Design review of the part built by this model. Coordinates are the model's own, in mm. A direction names the side the tool comes from. Coordinates: 2 decimals unless noted, no trailing zeros. Write each loop counter-clockwise with the first axis right and the second up, starting at its lowest first coordinate (ties: lowest second). Pieces come first, ordered by that corner, then holes.
```python
from build123d import *

# Parameters (mm, degrees)
F0_W     = 50.8
F0_H     = 50.8
F1_DEPTH = 76.2
F2_W     = 28.211626
F2_H     = 23.540352
F3_DEPTH = 94.742


with BuildPart() as f1:
    # F0 (on Top) → F1 (new body)
    with BuildSketch(Plane.XY):
        Rectangle(F0_W, F0_H)
    extrude(amount=F1_DEPTH)

    # F2 (on Top) → F3 (join)
    with BuildSketch(Plane.XY):
        with Locations((2.824979, 0)):
            Rectangle(F2_W, F2_H)
    extrude(amount=F3_DEPTH)


solid = f1.part
```
(1) Consider section C-C (z = 83.5). Give the boundary of the cut face in (x, y).
(2) Consider section A-A (x = 2.5). Give the boundary of the cut face in (y, z).
(3) Insertion check: pin 1 Ø8 at (x, z) = (-11.5, 81.5) entering from +Y; pin 2 Ø9.5 at (y, z) = (6, 84.5) entering from +X; pin 3 Ø6 at (x, y) = (9.5, 19.5) entering from -Z. Each pin has a flat end and moves straight along its axis. Give the tip position at first contact, or say it passes through.
(4) For faces 1 (the flat face through (-11.281, 0, 85)), 2 (the flat face through (16.931, 0, 85)), 3 (the flat face through (3, -11.77, 85)), list the 3-axis set-ups (+Z, -Z, +X, -X, +Y, -Y) from which the entire face can be reached by the end or side of a thin tool; tool diameter is ignored.
(5) Wall thickness on line 1 (Z direction, x = -13.5, y = -4); line 2 (X direction, y = 2.5, z = 79); line 3 (Y direction, x = -7, z = 84.5): over which ranges is each line inside the solid? List them lowest first.
(6) Consider section B-B (y = 6). Give the boundary of the cut face in (x, z), plus the area to 3 significant figures.
(7) Consider section D-D (x = -15). Give the boundary of the cut face in (y, z), plus the area to 3 significant figures.
Results:
1. outline: (-11.28, -11.77) - (16.93, -11.77) - (16.93, 11.77) - (-11.28, 11.77) - close
2. outline: (-25.4, 0) - (25.4, 0) - (25.4, 76.2) - (11.77, 76.2) - (11.77, 94.74) - (-11.77, 94.74) - (-11.77, 76.2) - (-25.4, 76.2) - close
3. pin 1: stops at y = 11.77
3. pin 2: stops at x = 16.93
3. pin 3: stops at z = 0
4. face 1: +Z, -X, +Y, -Y
4. face 2: +Z, +X, +Y, -Y
4. face 3: +Z, +X, -X, -Y
5. line 1: z = 0 to 76.2
5. line 2: x = -11.28 to 16.93
5. line 3: y = -11.77 to 11.77
6. outline: (-25.4, 0) - (25.4, 0) - (25.4, 76.2) - (16.93, 76.2) - (16.93, 94.74) - (-11.28, 94.74) - (-11.28, 76.2) - (-25.4, 76.2) - close
6. area: 4,390 mm2
7. outline: (-25.4, 0) - (25.4, 0) - (25.4, 76.2) - (-25.4, 76.2) - close
7. area: 3,870 mm2
